Could you check a few things on this model? Use its own coordinates, in mm. A direction names the side the tool comes from. Coordinates: 2 decimals unless noted, no trailing zeros. Loops run counter-clockwise (first coordinate to the right, second up) from the corner with the lowest first, then second, coordinate; pieces in that order, holes last.
1) Will these pins go through, and if not, where does the flat tip stop? P1, Ø4, axis at x = 34.5, z = 17, coming from the -Y side; P2, Ø4, axis at x = -30.5, y = -9, coming from the -Z side; P3, Ø1, axis at y = -7, z = 21.5, coming from the -X side; P4, Ø6, axis at x = -6.5, y = -6, coming from the -Z side.
2) Imagine slicing it at B-B on x = 11. Please give me the cut outline in (y, z).
3) Thinking about a two-plate mould opening in X: for faces 1 (the face through (-42.363, 1.268, -24.192)), 2 (the face through (42.363, 1.268, -24.192)), 3 (the face through (36.116, -0.74, 16.569)), which applies, released by +X, released by -X, zero draft, split by the parting line, or undercut?
4) For faces 4 (the face through (-8, -1.5, 18)), 5 (the face through (-37.5, -6, 22)), 6 (the face through (-21.5, -6, 22)), which set-ups out of +Z, -Z, +X, -X, +Y, -Y let a thin tool reach every point of the face, with its end or its side?
5) Imagine slicing it at A-A on y = -8.5. Give the number of separate pieces and of enclosed holes in the cut face, plus the area to 3 significant figures.
6) If I drill on line 1 along X through (y, z) = (-0.2, 17.51); line 2 along X through (y, z) = (-0.25, 1.61); line 3 along X through (y, z) = (2, 1.61), over which ranges is the centre line in solid material (lowest first)?
```python
from build123d import *

# Parameters (mm, degrees)
SKETCH1_W              = 91
SKETCH1_H              = 55
BOSS_EXTRUDE1_DEPTH    = 3.5
FILLET1_R              = 11
BOSS_EXTRUDE2_START    = -3.5
SKETCH2_W              = 10
SKETCH2_H              = 10
SKETCH2_W_2            = 8
SKETCH2_H_2            = 8
SKETCH2_W_3            = 4
SKETCH2_H_3            = 4
BOSS_EXTRUDE2_DEPTH    = 13
CUT_EXTRUDE1_START     = -10
SKETCH3_W              = 1
SKETCH3_H              = 3
SKETCH3_W_2            = 3
SKETCH3_H_2            = 1
CUT_EXTRUDE1_DEPTH     = 3
FILLET2_R              = 1.4999
LPATTERN1_COUNT        = 2
LPATTERN1_PITCH        = 15
FILLET2_OF_LPATTERN1_R = 1.4999
FILLET3_R              = 0.5
SKETCH4_R              = 1.75
SKETCH4_R_2            = 0.75
BOSS_EXTRUDE3_DEPTH    = 1.5
CUT_EXTRUDE2_START     = -3
SKETCH4_2_R            = 0.75
CUT_EXTRUDE2_DEPTH     = 3
FILLET4_R              = 1
SKETCH5_R              = 1.5
CUT_EXTRUDE3_DEPTH     = 55.731161166
SKETCH6_W              = 25.4
SKETCH6_H              = 31.75
CUT_EXTRUDE4_DEPTH     = 3
FILLET5_R              = 0.5
FILLET6_R              = 1


with BuildPart() as part:
    # Sketch1 → Boss-Extrude1 (new body)
    with BuildSketch(Plane(origin=(0, 0, 0), x_dir=(1, 0, 0), z_dir=(0, 1, 0))):
        Rectangle(SKETCH1_W, SKETCH1_H)
    extrude(amount=BOSS_EXTRUDE1_DEPTH)

    # Fillet1
    fillet1_edges = [part.edges().sort_by_distance(p)[0] for p in [
        (-45.5, 1.75, -27.5),
        (45.5, 1.75, -27.5),
        (45.5, 1.75, 27.5),
        (-45.5, 1.75, 27.5),
    ]]
    fillet(fillet1_edges, radius=FILLET1_R)

    # Sketch2 → Boss-Extrude2 (add)
    # profile 1 of 2: a face of its own
    with BuildSketch(Plane(origin=(0, 3.5, 0), x_dir=(1, 0, 0), z_dir=(0, 1, 0)).offset(BOSS_EXTRUDE2_START)):
        with Locations((-32.5, -21.5)):
            Rectangle(SKETCH2_W, SKETCH2_H)
        with Locations((-32.5, -21.5)):
            Rectangle(SKETCH2_W_2, SKETCH2_H_2, mode=Mode.SUBTRACT)
    # profile 2 of 2: a face of its own
    with BuildSketch(Plane(origin=(0, 3.5, 0), x_dir=(1, 0, 0), z_dir=(0, 1, 0)).offset(BOSS_EXTRUDE2_START)):
        with Locations((-32.5, -21.5)):
            Rectangle(SKETCH2_W_3, SKETCH2_H_3)
    boss_extrude2 = extrude(amount=-BOSS_EXTRUDE2_DEPTH)

    # Sketch3 → Cut-Extrude1 (cut)
    with BuildSketch(Plane(origin=(0, -13, 0), x_dir=(-1, 0, 0), z_dir=(0, -1, 0)).offset(CUT_EXTRUDE1_START)):
        with Locations((37, -24)):
            Rectangle(SKETCH3_W, SKETCH3_H)
        with Locations((30, -26)):
            Rectangle(SKETCH3_W_2, SKETCH3_H_2)
    cut_extrude1 = extrude(amount=-CUT_EXTRUDE1_DEPTH, mode=Mode.SUBTRACT)

    # Fillet2
    fillet2_edges = [part.edges().sort_by_distance(p)[0] for p in [
        (-28.5, 0, 22),
        (-37, -3, 25.5),
        (-37, -3, 22.5),
        (-31.5, 0, 26),
        (-31.5, -3, 26),
        (-28.5, -3, 26),
    ]]
    fillet(fillet2_edges, radius=FILLET2_R)

    # LPattern1: Boss-Extrude2, Cut-Extrude1 ×2
    with Locations(*[(i * LPATTERN1_PITCH, 0, 0) for i in range(1, LPATTERN1_COUNT)]):
        add(boss_extrude2)
        add(cut_extrude1, mode=Mode.SUBTRACT)

    # Fillet2 of LPattern1
    fillet2_of_lpattern1_edges = [part.edges().sort_by_distance(p)[0] for p in [
        (-13.5, 0, 22),
        (-22, -3, 25.5),
        (-22, -3, 22.5),
        (-16.5, 0, 26),
        (-16.5, -3, 26),
        (-13.5, -3, 26),
    ]]
    fillet(fillet2_of_lpattern1_edges, radius=FILLET2_OF_LPATTERN1_R)

    # Fillet3
    fillet3_edges = [part.edges().sort_by_distance(p)[0] for p in [
        (-37.5, -6.5, 26.5),
    ]]
    fillet(fillet3_edges, radius=FILLET3_R)

    # Sketch4 → Boss-Extrude3 (add)
    # profile 1 of 4: a face of its own
    with BuildSketch(Plane.XZ):
        with Locations(Location((34.64, 1.61, 0), (0, 0, 270))):
            Circle(SKETCH4_R)
        with Locations(Location((34.64, 1.61, 0), (0, 0, 270))):
            Circle(SKETCH4_R_2, mode=Mode.SUBTRACT)
    # profile 2 of 4: a face of its own
    with BuildSketch(Plane.XZ):
        with Locations(Location((34.64, 17.51, 0), (0, 0, 270))):
            Circle(SKETCH4_R)
        with Locations(Location((34.64, 17.51, 0), (0, 0, 270))):
            Circle(SKETCH4_R_2, mode=Mode.SUBTRACT)
    # profile 3 of 4: a face of its own
    with BuildSketch(Plane.XZ):
        with Locations(Location((-6.86, 17.51, 0), (0, 0, 270))):
            Circle(SKETCH4_R)
        with Locations(Location((-6.86, 17.51, 0), (0, 0, 270))):
            Circle(SKETCH4_R_2, mode=Mode.SUBTRACT)
    # profile 4 of 4: a face of its own
    with BuildSketch(Plane.XZ):
        with Locations(Location((-6.86, 1.61, 0), (0, 0, 270))):
            Circle(SKETCH4_R)
        with Locations(Location((-6.86, 1.61, 0), (0, 0, 270))):
            Circle(SKETCH4_R_2, mode=Mode.SUBTRACT)
    extrude(amount=BOSS_EXTRUDE3_DEPTH)

    # Sketch4<2> → Cut-Extrude2 (cut)
    with BuildSketch(Plane.XZ.offset(CUT_EXTRUDE2_START)):
        with Locations(Location((-6.86, 1.61, 0), (0, 0, 270))):
            Circle(SKETCH4_2_R)
        with Locations(Location((-6.86, 17.51, 0), (0, 0, 270))):
            Circle(SKETCH4_2_R)
        with Locations(Location((34.64, 17.51, 0), (0, 0, 270))):
            Circle(SKETCH4_2_R)
        with Locations(Location((34.64, 1.61, 0), (0, 0, 270))):
            Circle(SKETCH4_2_R)
    extrude(amount=CUT_EXTRUDE2_DEPTH, mode=Mode.SUBTRACT)

    # Fillet4
    fillet4_edges = [part.edges().sort_by_distance(p)[0] for p in [
        (-33.24995, 0, 17.5),
        (-28.939310539, -0.439310539, 17.5),
        (-12.5, -6.5, 26.5),
        (-22.5, -6.5, 26.5),
        (-22.5, -6.5, 16.5),
        (-12.5, -6.5, 16.5),
        (-21.5, -6.5, 17.5),
        (-13.5, -7.24995, 17.5),
        (-13.5, -7.25005, 25.5),
        (-21.5, -7.25005, 25.5),
        (-19.5, -6.5, 23.5),
        (-19.5, -6.5, 19.5),
        (-15.5, -6.5, 19.5),
        (-15.5, -6.5, 23.5),
        (-18.24995, 0, 17.5),
        (-13.939310539, -0.439310539, 17.5),
        (-27.5, -6.5, 26.5),
        (-37.5, -6.5, 16.5),
        (-27.5, -6.5, 16.5),
        (-36.5, -6.5, 17.5),
        (-28.5, -7.24995, 17.5),
        (-28.5, -7.25005, 25.5),
        (-36.5, -7.25005, 25.5),
        (-34.5, -6.5, 23.5),
        (-34.5, -6.5, 19.5),
        (-30.5, -6.5, 19.5),
        (-30.5, -6.5, 23.5),
    ]]
    fillet(fillet4_edges, radius=FILLET4_R - 0.0001)  # a hair under: the kernel refuses the full size

    # Sketch5 → Cut-Extrude3 (cut, through all)
    with BuildSketch(Plane.XZ):
        with Locations(Location((-31.5, -19.25, 0), (0, 0, 270))):
            Circle(SKETCH5_R)
    extrude(amount=-CUT_EXTRUDE3_DEPTH, mode=Mode.SUBTRACT)

    # Sketch6 → Cut-Extrude4 (cut)
    with BuildSketch(Plane.XZ):
        with Locations((-25.2, -0.864526382)):
            Rectangle(SKETCH6_W, SKETCH6_H)
    extrude(amount=-CUT_EXTRUDE4_DEPTH, mode=Mode.SUBTRACT)

    # Fillet5
    fillet5_edges = [part.edges().sort_by_distance(p)[0] for p in [
        (-37.9, 3, -0.864526382),
        (-25.2, 3, 15.010473618),
        (-12.5, 3, -0.864526382),
        (-25.2, 3, -16.739526382),
    ]]
    fillet(fillet5_edges, radius=FILLET5_R)

    # Fillet6
    fillet6_edges = [part.edges().sort_by_distance(p)[0] for p in [
        (0, 3.5, 27.5),
        (-45.5, 3.5, 0),
        (45.5, 3.5, 0),
        (0, 3.5, -27.5),
        (42.278174593, 3.5, 24.278174593),
        (42.278174593, 3.5, -24.278174593),
        (-42.278174593, 3.5, -24.278174593),
        (-42.278174593, 3.5, 24.278174593),
    ]]
    fillet(fillet6_edges, radius=FILLET6_R)


solid = part.part
```
Filled in:
1. P1: stops at y = -1.5
1. P2: stops at z = 16.5
1. P3: stops at x = -37.5
1. P4: passes through
2. outline: (0, -27.5) - (2.5, -27.5) arc R1 ccw to (3.5, -26.5) - (3.5, 26.5) arc R1 ccw to (2.5, 27.5) - (0, 27.5) - close
3. face 1: released by -X
3. face 2: released by +X
3. face 3: undercut
4. face 4: +Z, -Z, +X, -Y
4. face 5: +Z, -Z, -X, -Y
4. face 6: -Y
5. separate pieces: 4
5. enclosed holes: 2
5. area: 102 mm2
6. line 1: x = -37.5 to -27.5, -22.5 to -12.5, -8.61 to -7.61, -6.11 to -5.11, 32.89 to 33.89, 35.39 to 36.39
6. line 2: x = -8.61 to -7.61, -6.11 to -5.11, 32.89 to 33.89, 35.39 to 36.39
6. line 3: x = -45.5 to -37.9, -12.5 to -7.61, -6.11 to 33.89, 35.39 to 45.5
